CAD build for the part. Positions are in the model's coordinates, mm. Face numbers are marked on the shaded views. A direction names the side the tool comes from. Give positions to 0.01 mm unless a question says otherwise; leave off trailing zeros. Write each loop counter-clockwise with the first axis right and the second up, starting at its lowest first coordinate (ties: lowest second). Pieces come first, ordered by that corner, then holes. Notation, with made-up numbers: (-16.75, 40.25) - (23.25, 40.25) arc R6 ccw to (23.25, 49.25) - close; hole circle Ø1 at (-15.75, -4). An arc over 180 degrees is marked (long way). Write item = value, one per line. Start each with the question number.
```python
from build123d import *

# Parameters (mm, degrees)
SKETCH_1_W                                      = 42
SKETCH_1_H                                      = 42
EXTRUDE_1_DEPTH                                 = 17
CUT_EXTRUDE_1_DEPTH                             = 12.4
SKETCH_3_R                                      = 11.05
CUT_EXTRUDE_2_DEPTH                             = 8
SKETCH_5_R                                      = 1.2499999999999978
CUT_EXTRUDE_4_DEPTH                             = 12.4
FILLET_1_R                                      = 3
CHAMFER_1_SIZE                                  = 0.2
CHAMFER_2_SIZE                                  = 0.2
CHAMFER_3_SIZE                                  = 0.2
SKETCH_6_R                                      = 1.7500000000000004
SKETCH_6_R_2                                    = 1.7500000000000038
SKETCH_6_R_3                                    = 1.7499999999998814
SKETCH_6_R_4                                    = 1.7500000000000036
CUT_EXTRUDE_5_DEPTH                             = 26.00000000000001
CHAMFER_4_SIZE                                  = 0.2
FILETE2_R                                       = 3
CSK_FOR_M3_FLAT_HEAD_MACHINE_SCREW1_D           = 3.2
CSK_FOR_M3_FLAT_HEAD_MACHINE_SCREW1_CSINK_D     = 6.3
CSK_FOR_M3_FLAT_HEAD_MACHINE_SCREW1_CSINK_ANGLE = 90
TAP_DRILL_FOR_M6_TAP2_D                         = 5
TAP_DRILL_FOR_M6_TAP2_DEPTH                     = 6
TAP_DRILL_FOR_M6_TAP2_TIP                       = 1.5021515475689007


with BuildPart() as part:
    # Эскиз1 → Бобышка-Вытянуть1 (new body)
    with BuildSketch(Plane.XY):
        with Locations((21, 21)):
            Rectangle(SKETCH_1_W, SKETCH_1_H)
    extrude(amount=EXTRUDE_1_DEPTH)

    # Эскиз2 → Вырез-Вытянуть1 (cut)
    with BuildSketch(Plane.XY.offset(17)):
        with BuildLine():
            Line((0, 42), (42, 42))
            Line((42, 42), (42, 9.5))
            Line((42, 9.5), (21, 9.500000000000002))
            Line((21, 9.500000000000002), (21.00000000000009, 15.300000000000002))
            ThreePointArc((21.00000000000009, 15.300000000000002), (18.03693259362455, 16.130684694407922), (15.937505447941907, 18.380620510430074))
            Line((15.937505447941907, 18.380620510430074), (15.062505447941906, 18.380620510430074))
            ThreePointArc((15.062505447941906, 18.380620510430074), (12.29651275010685, 15.330331791538338), (8.337052317912484, 14.200000000000001))
            Line((8.337052317912484, 14.200000000000001), (8.337052317912484, 9.500000000000002))
            Line((8.337052317912484, 9.500000000000002), (3.98e-15, 9.500000000000002))
            Line((3.98e-15, 9.500000000000002), (0, 42))
        make_face()
    extrude(amount=-CUT_EXTRUDE_1_DEPTH, mode=Mode.SUBTRACT)

    # Эскиз3 → Вырез-Вытянуть2 (cut)
    with BuildSketch(Plane(origin=(0, 0, 0), x_dir=(-1, 0, 0), z_dir=(0, 0, -1))):
        with Locations((-21.000000000000007, 21.000000000000007)):
            Circle(SKETCH_3_R)
    extrude(amount=-CUT_EXTRUDE_2_DEPTH, mode=Mode.SUBTRACT)

    # Вырез-Вытянуть3 cone 1 section (through the dimple's axis) → Вырез-Вытянуть3 (revolve, cut)
    with BuildSketch(Plane(origin=(15, 18.38062051, 11.6), x_dir=(0, 0, 1), z_dir=(1, 0, 0))):
        Polygon((0, 0), (2.5, 0), (0, 20.36086607), align=None)
    revolve(axis=Axis((15, 18.38062051, 11.6), (0, -1, 0)), mode=Mode.SUBTRACT)

    # Эскиз5 → Вырез-Вытянуть4 (cut)
    with BuildSketch(Plane(origin=(0, 9.500000000000002, 0), x_dir=(1, -4e-17, 0), z_dir=(4e-17, 1, 0))):
        with Locations(Location((32.000000000000156, -10.600000000000055, 0), (0, 0, 180))):
            Circle(SKETCH_5_R)
    extrude(amount=-CUT_EXTRUDE_4_DEPTH, mode=Mode.SUBTRACT)

    # Скругление1
    # the kernel refuses this fillet: 3 mm, written as the material it adds along each edge
    with BuildSketch(Plane(origin=(21, 9.500000000000002, 17), x_dir=(1.54e-14, 1, 0), z_dir=(0, 0, -1))) as fillet_1_piece_1_section:
        with BuildLine():
            CenterArc((FILLET_1_R, FILLET_1_R), FILLET_1_R, 179.99999999999915, 90.00000000000085)
            Line((4.619e-14, FILLET_1_R), (0, 0))
            Line((0, 0), (FILLET_1_R, 0))
        make_face()
    fillet_1_piece_1 = extrude(amount=19.90000000000012, mode=Mode.PRIVATE)
    fillet_1_piece_1 = split(fillet_1_piece_1, bisect_by=Plane(origin=(21.37770329651456, 10.574866631857306, 8), z_dir=(0, 0, 1)), keep=Keep.TOP, mode=Mode.PRIVATE)
    add(fillet_1_piece_1)
    with BuildSketch(Plane(origin=(21, 9.500000000000002, 24.50000000000012), x_dir=(1.54e-14, 1, 0), z_dir=(0, 0, -1))) as fillet_1_piece_2_section:
        with BuildLine():
            CenterArc((FILLET_1_R, FILLET_1_R), FILLET_1_R, 179.99999999999915, 90.00000000000085)
            Line((4.619e-14, FILLET_1_R), (0, 0))
            Line((0, 0), (FILLET_1_R, 0))
        make_face()
    fillet_1_piece_2 = extrude(amount=19.90000000000012, mode=Mode.PRIVATE)
    fillet_1_piece_2 = fillet_1_piece_2 - Plane(origin=(21.000000000000007, 21.000000000000007, 6.3), x_dir=(-1, 0, 0), z_dir=(0, 0, -1)) * Cylinder(11.05, 52, mode=Mode.PRIVATE)
    fillet_1_piece_2 = split(fillet_1_piece_2, bisect_by=Plane(origin=(22.000979850131504, 9.712080299946667, 8), z_dir=(0, 0, -1)), keep=Keep.TOP, mode=Mode.PRIVATE)
    add(fillet_1_piece_2)
    with BuildSketch(Plane(origin=(8.337052317912484, 9.500000000000002, 17), x_dir=(-1, 0, 0), z_dir=(0, 0, -1))) as fillet_1_piece_3:
        with BuildLine():
            CenterArc((FILLET_1_R, FILLET_1_R), FILLET_1_R, 180, 90)
            Line((0, FILLET_1_R), (0, 0))
            Line((0, 0), (FILLET_1_R, 0))
        make_face()
    extrude(amount=12.4)
    # the kernel refuses this fillet: 3 mm, written as the material it takes off along each edge
    with BuildSketch(Plane(origin=(42, 42, -7.5), x_dir=(-1, 0, 0), z_dir=(0, 0, 1))) as fillet_1_2_piece_1:
        with BuildLine():
            CenterArc((FILLET_1_R, FILLET_1_R), FILLET_1_R, 180, 90)
            Line((0, FILLET_1_R), (0, 0))
            Line((0, 0), (FILLET_1_R, 0))
        make_face()
    extrude(amount=19.6, mode=Mode.SUBTRACT)
    with BuildSketch(Plane(origin=(0, 42, -7.5), x_dir=(1, 0, 0), z_dir=(0, 0, 1))) as fillet_1_2_piece_2:
        with BuildLine():
            CenterArc((FILLET_1_R, -FILLET_1_R), FILLET_1_R, 90, 90)
            Line((0, -FILLET_1_R), (0, 0))
            Line((0, 0), (FILLET_1_R, 0))
        make_face()
    extrude(amount=19.6, mode=Mode.SUBTRACT)
    with BuildSketch(Plane(origin=(42, 0, -7.5), x_dir=(-1, 0, 0), z_dir=(0, 0, 1))) as fillet_1_2_piece_3:
        with BuildLine():
            CenterArc((FILLET_1_R, -FILLET_1_R), FILLET_1_R, 90, 90)
            Line((0, -FILLET_1_R), (0, 0))
            Line((0, 0), (FILLET_1_R, 0))
        make_face()
    extrude(amount=32, mode=Mode.SUBTRACT)
    with BuildSketch(Plane(origin=(0, 0, -7.5), x_dir=(1, 0, 0), z_dir=(0, 0, 1))) as fillet_1_2_piece_4:
        with BuildLine():
            CenterArc((FILLET_1_R, FILLET_1_R), FILLET_1_R, 180, 90)
            Line((-4.4e-16, FILLET_1_R), (0, 0))
            Line((0, 0), (FILLET_1_R, 0))
        make_face()
    extrude(amount=32, mode=Mode.SUBTRACT)
    with BuildSketch(Plane(origin=(0, 9.500000000000002, 24.5), x_dir=(1, 0, 0), z_dir=(0, 0, -1))) as fillet_1_2_piece_5:
        with BuildLine():
            CenterArc((FILLET_1_R, FILLET_1_R), FILLET_1_R, 179.99999999999997, 90)
            Line((0, FILLET_1_R), (0, 0))
            Line((0, 0), (FILLET_1_R, 0))
        make_face()
    extrude(amount=19.900000000000006, mode=Mode.SUBTRACT)
    with BuildSketch(Plane(origin=(42, 9.5, 24.5), x_dir=(-1, 0, 0), z_dir=(0, 0, -1))) as fillet_1_2_piece_6:
        with BuildLine():
            CenterArc((FILLET_1_R, -FILLET_1_R), FILLET_1_R, 90, 90)
            Line((0, -FILLET_1_R), (0, 0))
            Line((0, 0), (FILLET_1_R, 0))
        make_face()
    extrude(amount=19.9, mode=Mode.SUBTRACT)

    # Фаска1
    chamfer_1_edges = [part.edges().sort_by_distance(p)[0] for p in [
        (32.05000000000001, 21.000000000000007, 0),
        (21, 42, 0),
        (0, 21, 0),
        (42, 21, 0),
        (21, 0, 0),
        (0.8786796564403576, 0.8786796564403572, 0),
        (41.121320343559645, 0.8786796564403576, 0),
        (0.8786796564403572, 41.121320343559645, 0),
        (41.121320343559645, 41.121320343559645, 0),
    ]]
    chamfer(chamfer_1_edges, length=CHAMFER_1_SIZE)

    # Фаска2
    chamfer_2_edges = [part.edges().sort_by_distance(p)[0] for p in [
        (42, 22.75, 4.6000000000000005),
        (12.296512750106848, 15.330331791538338, 17),
        (15.500005447941906, 18.380620510430074, 17),
        (18.036932593624567, 16.13068469440791, 17),
        (21.000000000000068, 13.900000000000002, 17),
        (31.500000000000014, 9.5, 17),
        (21, 42, 4.6),
        (9e-17, 22.75, 4.6000000000000005),
        (0.8786796564403572, 41.121320343559645, 4.6),
        (41.121320343559645, 41.121320343559645, 4.6),
        (8.337052317912484, 13.350000000000001, 17),
        (4.168526158956, 9.500000000000002, 17),
        (42, 4.75, 17),
        (0, 4.75, 17),
        (21, 0, 17),
        (0.8786796564403576, 8.621320343559642, 17),
        (0.8786796564403576, 0.8786796564403572, 17),
        (41.121320343559645, 8.621320343559642, 17),
        (41.121320343559645, 0.8786796564403576, 17),
        (21.878679656440376, 10.378679656440339, 17),
        (7.4583726614716435, 10.378679656440358, 17),
    ]]
    chamfer(chamfer_2_edges, length=CHAMFER_2_SIZE)

    # Фаска3
    chamfer_3_edges = [part.edges().sort_by_distance(p)[0] for p in [
        (28.33886931397383, 29.260962243734895, 4.6),
    ]]
    chamfer(chamfer_3_edges, length=CHAMFER_3_SIZE)

    # Эскиз6 → Вырез-Вытянуть5 (cut)
    with BuildSketch(Plane(origin=(0, 0, 0), x_dir=(-1, 0, 0), z_dir=(0, 0, -1))):
        with Locations((-5.50000000000014, 36.50000000000002)):
            Circle(SKETCH_6_R)
        with Locations((-36.50000000000014, 36.50000000000001)):
            Circle(SKETCH_6_R_2)
        with Locations((-5.500000000000008, 5.5000000000000115)):
            Circle(SKETCH_6_R_3)
        with Locations((-36.50000000000013, 5.500000000000008)):
            Circle(SKETCH_6_R_4)
    extrude(amount=-CUT_EXTRUDE_5_DEPTH, mode=Mode.SUBTRACT)

    # Фаска4
    chamfer_4_edges = [part.edges().sort_by_distance(p)[0] for p in [
        (7.25000000000014, 36.50000000000002, 4.6),
        (7.25000000000014, 36.50000000000002, 0),
        (38.25000000000015, 36.50000000000001, 4.6),
        (38.25000000000015, 36.50000000000001, 0),
        (7.24999999999989, 5.5000000000000115, 17),
        (7.24999999999989, 5.5000000000000115, 0),
        (38.25000000000013, 5.500000000000008, 17),
        (38.25000000000013, 5.500000000000008, 0),
    ]]
    chamfer(chamfer_4_edges, length=CHAMFER_4_SIZE)

    # Filete2
    filete2_edges = [part.edges().sort_by_distance(p)[0] for p in [
        (16.297005113109307, 11.000783075966405, 8),
    ]]
    fillet(filete2_edges, radius=FILETE2_R)

    # CSK for M3 Flat Head Machine Screw1 (through all)
    with Locations(Plane.XY.offset(4.600000000000001)):
        with Locations((36.5, 36.5)):
            CounterSinkHole(CSK_FOR_M3_FLAT_HEAD_MACHINE_SCREW1_D / 2, CSK_FOR_M3_FLAT_HEAD_MACHINE_SCREW1_CSINK_D / 2, counter_sink_angle=CSK_FOR_M3_FLAT_HEAD_MACHINE_SCREW1_CSINK_ANGLE)

    # Tap Drill for M6 Tap2
    with Locations(Plane(origin=(0, 0, 0), x_dir=(-1, 0, 0), z_dir=(0, -1, 0))):
        with Locations((-15, -11.6)):
            Hole(TAP_DRILL_FOR_M6_TAP2_D / 2, depth=TAP_DRILL_FOR_M6_TAP2_DEPTH)
            with Locations((0, 0, -(TAP_DRILL_FOR_M6_TAP2_DEPTH + TAP_DRILL_FOR_M6_TAP2_TIP / 2))):  # 118° drill point
                Cone(0, TAP_DRILL_FOR_M6_TAP2_D / 2, TAP_DRILL_FOR_M6_TAP2_TIP, mode=Mode.SUBTRACT)


solid = part.part
```
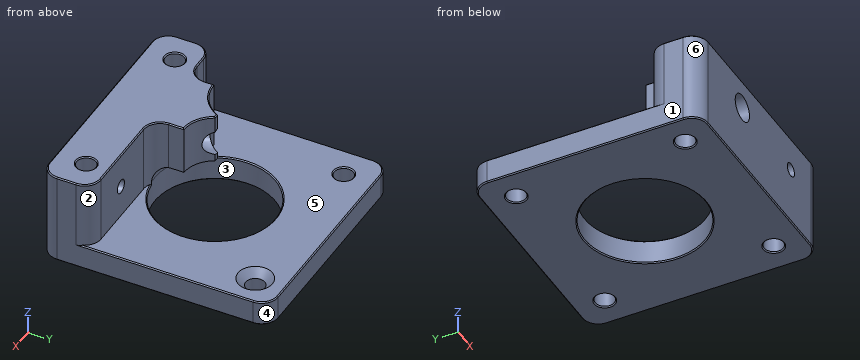
1. Tool access for the marked faces 1 and 2: list every direction of +Z, -Z, +X, -X, +Y, -Y with a clear straight run to the whole face (end or side of a thin tool).
2. Cut at C-C (z = 2). Give the cut face in (x, y), then the cut area to 3 significant figures.
3. Wall check: line 1 along Z through (x, y) = (32, 7); line 2 along Y through (x, z) = (5.5, 2.95); line 3 along Y through (x, z) = (21, 1.5). Give the ranges that are in metal, low to high.
4. Cut at A-A (x = 36.5). Give the cut face in (y, z), then the cut area to 3 significant figures.
5. Pin check, flat tips, straight feed: pin 1 Ø3 at (x, y) = (5.5, 36.5) entering from -Z; pin 2 Ø0.5 at (y, z) = (13.5, 12) entering from -X; pin 3 Ø1.6 at (x, y) = (17.5, 16) entering from -Z; pin 4 Ø3 at (x, z) = (32, 10.6) entering from +Y. Stop position of each tip, or through.
6. Mould opens along Y. For the marked faces 3, 4, 5 and 6 say: +Y half, -Y half, draft (parallel to the pull), parting line (faces both ways), or undercut.
7. Cut at B-B (y = 5.5). Give the cut face in (x, z).
8. Cut at D-D (z = 8.5). Give the cut face in (x, y), then the cut area to 3 significant figures.
Output:
q1.face_1 = +Z, -Z, -X, +Y, -Y
q1.face_2 = +Z, +X, +Y
q2.outline = (0, 3) arc R3 ccw to (3, 0) - (39, 0) arc R3 ccw to (42, 3) - (42, 39) arc R3 ccw to (39, 42) - (3, 42) arc R3 ccw to (0, 39) - close; hole circle Ø3.5 at (5.5, 5.5); hole circle Ø3.5 at (5.5, 36.5); hole circle Ø22.1 at (21, 21); hole circle Ø3.5 at (36.5, 5.5); hole circle Ø3.5 at (36.5, 36.5)
q2.area = 1,330 mm2
q3.line_1 = 0 to 9.35, 11.85 to 17
q3.line_2 = 0 to 3.75, 7.25 to 34.75, 38.25 to 42
q3.line_3 = 0 to 9.95, 32.05 to 42
q4.outline = (0, 0.2) - (0.2, 0) - (3.55, 0) - (3.75, 0.2) - (3.75, 16.8) - (3.55, 17) - (0.2, 17) - (0, 16.8) - close; (7.25, 0.2) - (7.45, 0) - (34.55, 0) - (34.75, 0.2) - (34.75, 3.2) - (33.35, 4.6) - (9.5, 4.6) - (9.5, 16.8) - (9.3, 17) - (7.45, 17) - (7.25, 16.8) - close; (38.25, 0.2) - (38.45, 0) - (41.8, 0) - (42, 0.2) - (42, 4.4) - (41.8, 4.6) - (39.65, 4.6) - (38.25, 3.2) - close
q4.area = 233 mm2
q5.pin_1 = through
q5.pin_2 = 8.34
q5.pin_3 = 8
q5.pin_4 = 9.5
q6.face_3 = undercut
q6.face_4 = +Y half
q6.face_5 = draft
q6.face_6 = -Y half
q7.outline = (0, 0.2) - (0.2, 0) - (3.55, 0) - (3.75, 0.2) - (3.75, 16.8) - (3.55, 17) - (0.2, 17) - (0, 16.8) - close; (7.25, 0.2) - (7.45, 0) - (34.55, 0) - (34.75, 0.2) - (34.75, 16.8) - (34.55, 17) - (7.45, 17) - (7.25, 16.8) - close; (38.25, 0.2) - (38.45, 0) - (41.8, 0) - (42, 0.2) - (42, 16.8) - (41.8, 17) - (38.45, 17) - (38.25, 16.8) - close; hole circle Ø5 at (15, 11.6); hole circle Ø2.5 at (32, 10.6)
q8.outline = (0, 3) arc R3 ccw to (3, 0) - (39, 0) arc R3 ccw to (42, 3) - (42, 6.5) arc R3 ccw to (39, 9.5) - (24, 9.5) arc R3 cw to (21, 12.5) - (21, 15.3) arc R5.7 cw to (15.94, 18.38) - (15.06, 18.38) arc R7.5 cw to (8.34, 14.2) - (8.34, 12.5) arc R3 cw to (5.34, 9.5) - (3, 9.5) arc R3 ccw to (0, 6.5) - close; hole circle Ø3.5 at (5.5, 5.5); hole circle Ø3.5 at (36.5, 5.5)
q8.area = 457 mm2
